Check sheet for the modelled part. Datum: model origin and axes. Units: mm. Face numbers are marked on the shaded views. A direction names the side the tool comes from. Coordinates: 2 decimals unless noted, no trailing zeros. Loops run counter-clockwise (first coordinate to the right, second up) from the corner with the lowest first, then second, coordinate; pieces in that order, holes last. Notation, with made-up numbers: (37.5, -13.75) - (43.5, -13.75) arc R22 cw to (43.5, 21.25) - close; hole circle Ø7 at (0, 38.5). An arc over 180 degrees is marked (long way). Answer as a JSON object with one key per item and string values. Group by question number.
Autodesk Inventor part; units mm, degrees
ref_plane "Work Plane4" through (-17.3656, 0.1134, 28.8) normal (-1, 0, 0) x (0, 0, 1)
ref_plane "YZ Plane" through (0, 0, 0) normal (1, 0, 0) x (0, 1, 0)
ref_plane "XZ Plane" through (0, 0, 0) normal (0, 1, 0) x (-1, 0, 0)
sketch "Sketch1" plane through (0, 0, 0) normal (0, 0, 1) x (1, 0, 0)
  line L0 (-17.3656, -3.1866) -> (12.6344, -3.1866)
  line L1 (12.6344, -3.1866) -> (12.6344, 9.8134)
  line L2 (12.6344, 9.8134) -> (-17.3656, 9.8134)
  line L3 (-17.3656, 9.8134) -> (-17.3656, -3.1866)
  point P0 (0, 0)
  dimension "d0" = 30
  dimension "d1" = 13
extrude "Extrusion1" add sketch "Sketch1" along normal blind 35
sketch "Sketch2" plane through (0, 0, 35) normal (0, 0, 1) x (1, 0, 0)
  point P0 (0, 0)
sketch "Sketch3" plane through (0, 0, 35) normal (0, 0, 1) x (1, 0, 0)
  line L0 (-24.8388, 28.6624) -> (-24.5328, 28.6624)
  line L1 (12.6344, -3.1866) -> (12.6344, 9.8134)
  line L2 (-17.3656, 9.8134) -> (-17.3656, -3.1866)
  line L3 (-17.3656, 11.3273) -> (-17.3656, 4.8273)
  line L4 (15.1579, 11.3273) -> (15.1579, 4.8273)
  line L5 (-17.3656, 4.8273) -> (15.1579, 4.8273)
  line L6 (-17.3656, 11.3273) -> (15.1579, 11.3273)
  line L7 (-43.7964, 23.1681) -> (-44.8479, 23.9265)
  line L8 (-44.8479, 23.9265) -> (-43.7964, 23.1681)
  line L9 (-42.6813, 23.9265) -> (-43.7964, 23.1681)
  line L10 (-44.8479, 23.9265) -> (-45.923, 23.1739)
  line L11 (-41.5979, 23.1681) -> (-42.6813, 23.9265)
  line L12 (-40.5146, 23.9265) -> (-41.5979, 23.1681)
  line L13 (-38.3479, 23.9265) -> (-37.2646, 23.1681)
  line L14 (-37.2646, 23.1681) -> (-38.3479, 23.9265)
  line L15 (-40.5146, 23.9265) -> (-39.4313, 23.1681)
  line L16 (-38.3479, 23.9265) -> (-39.4313, 23.1681)
  line L17 (-39.4313, 23.1681) -> (-40.5146, 23.9265)
  line L18 (-30.7646, 23.1681) -> (-29.6813, 23.9265)
  line L19 (-29.6813, 23.9265) -> (-30.7646, 23.1681)
  line L20 (-31.8479, 23.9265) -> (-30.7646, 23.1681)
  line L21 (-32.9313, 23.1681) -> (-31.8479, 23.9265)
  line L22 (-36.1813, 23.9265) -> (-35.0979, 23.1681)
  line L23 (-34.0146, 23.9265) -> (-35.0979, 23.1681)
  line L24 (-35.0979, 23.1681) -> (-34.0146, 23.9265)
  line L25 (-34.0146, 23.9265) -> (-32.9313, 23.1681)
  line L26 (-36.1813, 23.9265) -> (-37.2646, 23.1681)
  line L27 (-29.6813, 23.9265) -> (-28.5979, 23.1681)
  line L28 (-14.5146, 23.9265) -> (-13.3995, 23.1739)
  line L29 (-15.5979, 23.1681) -> (-14.5146, 23.9265)
  line L30 (-16.6813, 23.9265) -> (-15.5979, 23.1681)
  line L31 (-16.6813, 23.9265) -> (-17.7646, 23.1681)
  line L32 (-17.7646, 23.1681) -> (-16.6813, 23.9265)
  line L33 (-18.8479, 23.9265) -> (-17.7646, 23.1681)
  line L34 (-18.8479, 23.9265) -> (-19.9313, 23.1681)
  line L35 (-19.9313, 23.1681) -> (-18.8479, 23.9265)
  line L36 (-21.0146, 23.9265) -> (-19.9313, 23.1681)
  line L37 (-21.0146, 23.9265) -> (-22.0979, 23.1681)
  line L38 (-23.1813, 23.9265) -> (-22.0979, 23.1681)
  line L39 (-22.0979, 23.1681) -> (-23.1813, 23.9265)
  line L40 (-23.1813, 23.9265) -> (-24.2646, 23.1681)
  line L41 (-24.2646, 23.1681) -> (-25.3479, 23.9265)
  line L42 (-26.4313, 23.1681) -> (-27.5146, 23.9265)
  line L43 (-27.5146, 23.9265) -> (-26.4313, 23.1681)
  line L44 (-25.3479, 23.9265) -> (-26.4313, 23.1681)
  line L45 (-27.5146, 23.9265) -> (-28.5979, 23.1681)
  line L46 (-45.923, 23.1739) -> (-45.923, 16.6739)
  line L47 (-13.3995, 23.1739) -> (-13.3995, 16.6739)
  line L48 (-45.923, 16.6739) -> (-13.3995, 16.6739)
  line L49 (-45.923, 23.1739) -> (-13.3995, 23.1739)
  point P0 (-17.3656, 7.8134)
  point P1 (10.6344, 9.8134)
  point P2 (-15.3656, 9.8134)
  point P3 (-17.3656, 2.7291)
  point P4 (15.1344, 5.7756)
  point P5 (-17.3656, 5.5444)
  point P6 (-17.3656, 2.7304)
  point P7 (12.6344, 4.8273)
  point P8 (-17.3656, 9.8134)
  point P9 (-45.923, 19.66)
  point P10 (-17.923, 21.66)
  point P11 (-43.923, 21.66)
  point P12 (-45.923, 21.66)
  point P13 (-15.923, 21.66)
  point P14 (-37.2646, 23.1828)
  point P15 (-19.9313, 23.1828)
  point P16 (-45.923, 17.391)
  dimension "d79" = 6.5
fillet "Fillet2" radius 2 2 edges at (-17.3656, -3.1866, 17.5) (12.6344, -3.1866, 17.5)
sketch "Sketch5" plane through (0, 0, 35) normal (0, 0, 1) x (1, 0, 0)
  line L0 (-17.3656, 0.1134) -> (-17.3656, 5.1134)
  line L1 (-17.3656, 21.8134) -> (-17.3656, 25.9634) construction
  line L2 (12.6344, 9.8134) -> (-17.3656, 9.8134) construction
  line L3 (-17.3656, 44.8134) -> (12.6344, 44.8134)
  line L4 (12.6344, 21.8134) -> (12.6344, 44.8134)
  line L5 (-17.3656, 9.8134) -> (12.6344, 9.8134) construction
  line L6 (-17.3656, 21.8134) -> (-17.3656, 44.8134)
  line L7 (12.6344, 9.8134) -> (-17.3656, 9.8134)
  line L8 (-17.3656, 21.8134) -> (-17.3656, 9.8134)
  line L9 (12.6344, 21.8134) -> (12.6344, 9.8134)
  line L10 (12.6344, 9.8134) -> (2.6344, 9.8134)
  point P0 (0, 0)
  point P1 (-17.3656, 2.6134)
  dimension "d15" = 23.35
  dimension "d17" = 35
  dimension "d20" = 30
  dimension "d21" = 10
extrude "Extrusion4" add sketch "Sketch5" against normal blind 35
ref_plane "Work Plane4" through (-17.3656, 0.1134, 28.8) normal (-1, 0, 0) x (0, 0, 1)
sketch "Sketch6" plane through (-17.3656, 0.1134, 28.8) normal (-1, 0, 0) x (0, 0, 1)
  line L0 (6.2, 44.7) -> (6.2, 5)
  line L1 (6.2, 29.7) -> (-11.3, 29.7) construction
  line L2 (6.2, 29.7) -> (23.7, 29.7) construction
  circle A0 centre (-11.3, 29.7) radius 11.1
  line L3 (6.2, 44.7) -> (-28.8, 44.7)
  point P0 (-28.8, -0.1134)
  point P1 (6.2, 27.7)
  dimension "d24" = 17.5
  dimension "d25" = 180
  dimension "d26" = 22.2
  dimension "d58" = 15
fillet "Fillet3" radius 2 2 edges at (-17.3656, 44.8134, 17.5) (12.6344, 44.8134, 17.5)
extrude "Extrusion7" cut sketch "Sketch6" against normal blind 35
sketch "Sketch8" plane through (0, 0, 0) normal (0, 0, -1) x (-1, 0, 0)
  circle A0 centre (-4.6344, 11.0711) radius 1.5
  circle A1 centre (-4.6344, 11.0711) radius 1.5
  circle A2 centre (-4.6344, 16.0711) radius 1.5
  circle A3 centre (-4.6344, 16.0711) radius 1.5
  circle A4 centre (9.3656, 16.0711) radius 1.5
  circle A5 centre (9.3656, 16.0711) radius 1.5
  circle A6 centre (9.3656, 11.0711) radius 1.5
  circle A7 centre (9.3656, 11.0711) radius 1.5
  point P0 (0, 0)
extrude "Extrusion8" cut sketch "Sketch8" against normal blind 10
sketch "Sketch9" plane through (0, 0, 35) normal (0, 0, 1) x (1, 0, 0)
  point P0 (0, 0)
extrude "Extrusion14" cut sketch "Sketch3" against normal blind 30 contours L3 L6 L4 L5 L2
thread "Thread1"
thread "Thread2"
thread "Thread3"
thread "Thread4"
properties part number "Beltclamp"
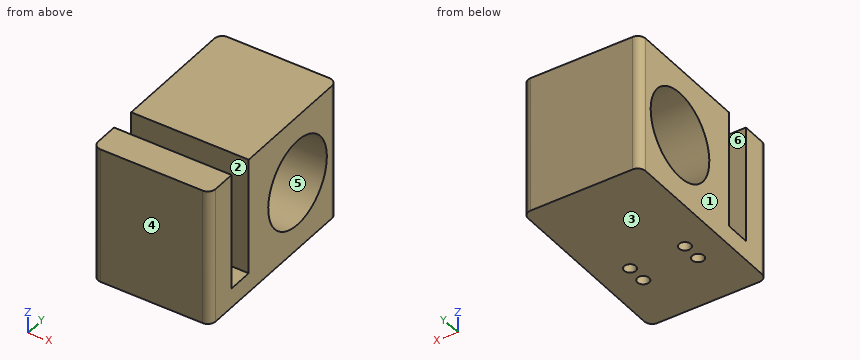
1. Gauge pin test, flat ends, axial feed: pin 1 (1.4 mm diameter, centred on x = -9.5, y = 11.5, fed in from -Z); pin 2 (1.9 mm diameter, centred on x = -2, y = 9.5, fed in from +Z). Record the tip position at first contact, or that the pin passes through.
2. Access from +Z, -Z, +X, -X, +Y, -Y to the whole of each face (thin tool, end or side, straight path). Record for the marked faces 1 and 2.
3. Sectioned sample at C-C on y = 37.5. Record the cut outline in (x, z), plus the area to 3 significant figures.
4. Release check for a two-part mould opening along Y. For the marked faces 3, 4, 5 and 6 record: released by +Y, released by -Y, zero draft, split by the parting line, or undercut.
5. Sectioned sample at A-A on x = -8.75. Record the cut outline in (y, z), plus the area to 3 significant figures.
6. Material ranges on line 1 (Y direction, x = -10, z = 29.5); line 2 (Y direction, x = 5.75, z = 3); line 3 (Y direction, x = 3.5, z = 25), recorded low to high.
7. Sectioned sample at D-D on z = 31. Record the cut outline in (x, y), plus the area to 3 significant figures.
8. Sectioned sample at B-B on z = 13. Record the cut outline in (x, y), plus the area to 3 significant figures.
Answers follow:
{
 "1": {"pin 1": "stops at z = 10", "pin 2": "stops at z = 5"},
 "2": {"face 1": "+Z, -Z, -X, +Y, -Y", "face 2": "+Z, +X, -X"},
 "3": {"outline": "(-17.37, 0) - (12.63, 0) - (12.63, 9.49) - (-17.37, 9.49) - close; (-17.37, 25.51) - (12.63, 25.51) - (12.63, 35) - (-17.37, 35) - close", "area": "570 mm^2"},
 "4": {"face 3": "zero draft", "face 4": "released by -Y", "face 5": "undercut", "face 6": "undercut"},
 "5": {"outline": "(-3.19, 0) - (9.7, 0) - (9.7, 5) - (4.83, 5) - (4.83, 35) - (-3.19, 35) - close; (11.33, 10) - (12.44, 10) - (12.44, 0) - (14.7, 0) - (14.7, 10) - (17.44, 10) - (17.44, 0) - (44.81, 0) - (44.81, 35) - (11.33, 35) - close; hole circle Ø22.2 at (29.81, 17.5)", "area": "1,050 mm^2"},
 "6": {"line 1": "y = -3.19 to 4.83, 11.33 to 44.81", "line 2": "y = -3.19 to 10.07, 12.07 to 15.07, 17.07 to 44.81", "line 3": "y = -3.19 to 4.83, 11.33 to 21.63, 38 to 44.81"},
 "7": {"outline": "(-17.37, -1.19) arc R2 ccw to (-15.37, -3.19) - (10.63, -3.19) arc R2 ccw to (12.63, -1.19) - (12.63, 4.83) - (-17.37, 4.83) - close; (-17.37, 11.33) - (12.63, 11.33) - (12.63, 42.81) arc R2 ccw to (10.63, 44.81) - (-15.37, 44.81) arc R2 ccw to (-17.37, 42.81) - close", "area": "1,240 mm^2"},
 "8": {"outline": "(-17.37, -1.19) arc R2 ccw to (-15.37, -3.19) - (10.63, -3.19) arc R2 ccw to (12.63, -1.19) - (12.63, 4.83) - (-17.37, 4.83) - close; (-17.37, 11.33) - (12.63, 11.33) - (12.63, 19.67) - (-17.37, 19.67) - close; (-17.37, 39.96) - (12.63, 39.96) - (12.63, 42.81) arc R2 ccw to (10.63, 44.81) - (-15.37, 44.81) arc R2 ccw to (-17.37, 42.81) - close", "area": "633 mm^2"}
}
